Input: dimensioned drawing with shaded views. Units: mm. Origin: part minimum x, y, z. A direction names the side the tool comes from. Round coordinates to 2 decimals unless told otherwise and drop trailing zeros. Order: outer loops, then holes, each group sorted by start corner. A loop starts at its lowest first (then second) coordinate and runs counter-clockwise, first axis right, second up. Notation, with made-up numbers: (73.25, 30) - (110.25, 30) arc R27 cw to (110.25, 51) - close; hole circle Ø8 at (61.25, 19). An arc over 180 degrees is marked (long way). Return JSON: item names as keys, results as strings. Group by question number.
1) Ray query, line 1 (Y direction, x = 15, z = 3); line 2 (Y direction, x = 16.25, z = 7); line 3 (Z direction, x = 11.25, y = 19). Return the intervals inside material, ascending. Write a range as from..to.
2) Section C-C, the plane y = 18.5. Return loops of the section in (x, z).
3) Section B-B, the plane x = 6. Return loops of the section in (y, z).
4) Contact query for flat-ended pins moving along their axis: P1, Ø3, axis at y = 12, z = 37, coming from the -X side; P2, Ø4.5, axis at y = 12, z = 38.5, coming from the +X side; P3, Ø10, axis at y = 19, z = 15, coming from the -X side. Output: stop coordinate, or through.
5) Section D-D, the plane x = 12.5. Return loops of the section in (y, z).
6) Mould query, pull axis X, two halves, no side actions, for the marked faces 1, 2, 3 and 4. Classes: pulls with the +X half, pulls with the -X half, needs draft (parallel to the pull), parting line crosses it, or undercut.
7) Access query for the marked faces 5, 6 and 7. Directions: +Z, -Z, +X, -X, +Y, -Y. A direction counts if a zero-diameter tool reaches every point of the face in a straight line with its end or side. Return the directions, or none.
8) Section A-A, the plane z = 23. Return loops of the section in (x, y), plus the area to 3 significant figures.
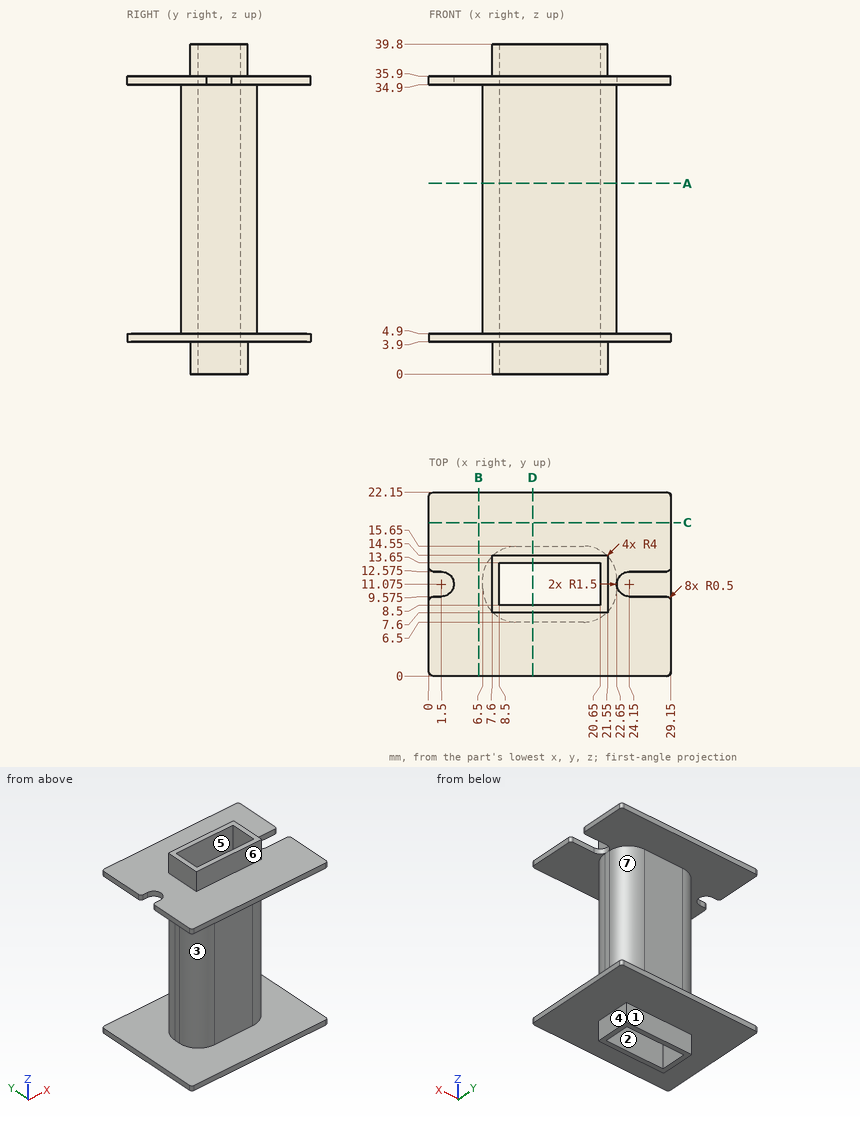
Geometry check:
{
 "1": {"line 1": "7.6..8.5, 13.65..14.55", "line 2": "6.5..8.5, 13.65..15.65", "line 3": "3.9..4.9, 34.9..35.9"},
 "2": {"outline": "(0, 3.9) - (29.15, 3.9) - (29.15, 4.9) - (0, 4.9) - close; (0, 34.9) - (29.15, 34.9) - (29.15, 35.9) - (0, 35.9) - close"},
 "3": {"outline": "(0, 3.9) - (22.15, 3.9) - (22.15, 4.9) - (0, 4.9) - close; (0, 34.9) - (22.15, 34.9) - (22.15, 35.9) - (0, 35.9) - close"},
 "4": {"P1": "x = 0", "P2": "x = 21.55", "P3": "x = 7.26"},
 "5": {"outline": "(0, 3.9) - (7.6, 3.9) - (7.6, 0) - (8.5, 0) - (8.5, 39.8) - (7.6, 39.8) - (7.6, 35.9) - (0, 35.9) - (0, 34.9) - (6.5, 34.9) - (6.5, 4.9) - (0, 4.9) - close; (13.65, 0) - (14.55, 0) - (14.55, 3.9) - (22.15, 3.9) - (22.15, 4.9) - (15.65, 4.9) - (15.65, 34.9) - (22.15, 34.9) - (22.15, 35.9) - (14.55, 35.9) - (14.55, 39.8) - (13.65, 39.8) - close"},
 "6": {"face 1": "needs draft", "face 2": "undercut", "face 3": "pulls with the -X half", "face 4": "pulls with the +X half"},
 "7": {"face 5": "+Z, -Z", "face 6": "+Z, +X, -X, -Y", "face 7": "+X, +Y"},
 "8": {"outline": "(6.5, 10.5) arc R4 ccw to (10.5, 6.5) - (18.65, 6.5) arc R4 ccw to (22.65, 10.5) - (22.65, 11.65) arc R4 ccw to (18.65, 15.65) - (10.5, 15.65) arc R4 ccw to (6.5, 11.65) - close; hole (8.5, 8.5) - (20.65, 8.5) - (20.65, 13.65) - (8.5, 13.65) - close", "area": "71.5 mm2"}
}
